Source: CAD feature listing. Evaluate the final solid. Frame: model axes, mm. A direction names the side the tool comes from. Give positions to 0.01 mm unless a question says otherwise; leave off trailing zeros. Loops run counter-clockwise (first coordinate to the right, second up) from the corner with the lowest first, then second, coordinate; pieces in that order, holes last. Notation, with made-up numbers: M -17.5,73.25 L 6.5,73.25 A19 cw 6.5,77.25 Z; hole C 7.5,-20.75 d10. An arc over 180 degrees is marked long. Answer in a Markdown table with one row per item.
```python
from build123d import *

# Parameters (mm, degrees)
SKETCH_3_W           = 180
SKETCH_3_H           = 43
EXTRUDE_1_DEPTH      = 12
CUT_EXTRUDE_1_DEPTH  = 52
CUT_EXTRUDE_2_DEPTH  = 5
CUT_EXTRUDE_3_DEPTH  = 5
SKETCH_8_W           = 55
SKETCH_8_H           = 37
CUT_EXTRUDE_4_DEPTH  = 10.5
CUT_EXTRUDE_5_DEPTH  = 4
SKETCH_10_W          = 62.128790526
SKETCH_10_H          = 8.683746703
CUT_EXTRUDE_6_DEPTH  = 8
CUT_EXTRUDE_8_DEPTH  = 9
FILLET_2_R           = 2
FILLET_3_R           = 3
SKETCH_12_W          = 10
SKETCH_12_H          = 4
CUT_EXTRUDE_9_DEPTH  = 10
SKETCH_13_W          = 4
SKETCH_13_H          = 4
SKETCH_13_H_2        = 7.435323836
SKETCH_13_W_2        = 5
SKETCH_13_H_3        = 5
EXTRUDE_2_DEPTH      = 5
SKETCH_14_W          = 15
SKETCH_14_H          = 1.5
CUT_EXTRUDE_10_DEPTH = 5.5


with BuildPart() as part:
    # 草图3 → 凸台-拉伸1 (new body)
    with BuildSketch(Plane(origin=(0, 0, 0), x_dir=(1, 0, 0), z_dir=(0, 1, 0))):
        with Locations((50.068597249, 7.753123643)):
            Rectangle(SKETCH_3_W, SKETCH_3_H)
    extrude(amount=EXTRUDE_1_DEPTH)

    # 草图4 → 切除-拉伸1 (cut)
    with BuildSketch(Plane(origin=(0, 0, 0), x_dir=(1, 0, 0), z_dir=(0, 1, 0))):
        Polygon((-22.469613434, -5.858946979), (26.002261286, -5.858946979), (29.068597249, -13.746876357), (-25.931402751, -13.746876357), align=None)
    extrude(amount=CUT_EXTRUDE_1_DEPTH, mode=Mode.SUBTRACT)

    # 草图5 → 切除-拉伸2 (cut)
    with BuildSketch(Plane(origin=(0, 12, 0), x_dir=(1, 0, 0), z_dir=(0, 1, 0))):
        Polygon((140.068597249, 7.753123643), (140.068597249, 22.753123643), (125.276479966, 22.753123643), (125.276479966, -7.246876357), (140.068597249, -7.246876357), align=None)
    extrude(amount=-CUT_EXTRUDE_2_DEPTH, mode=Mode.SUBTRACT)

    # 草图7 → 切除-拉伸3 (cut)
    with BuildSketch(Plane(origin=(0, 12, 0), x_dir=(1, 0, 0), z_dir=(0, 1, 0))):
        Polygon((125.276479966, 7.753123643), (125.276479966, 25.753123643), (100.500825538, 25.753123643), (100.500825538, -10.246876357), (125.276479966, -10.246876357), align=None)
    extrude(amount=-CUT_EXTRUDE_3_DEPTH, mode=Mode.SUBTRACT)

    # 草图8 → 切除-拉伸4 (cut)
    with BuildSketch(Plane(origin=(0, 12, 0), x_dir=(1, 0, 0), z_dir=(0, 1, 0))):
        with Locations((63.776287419, 7.753123643)):
            Rectangle(SKETCH_8_W, SKETCH_8_H)
    extrude(amount=-CUT_EXTRUDE_4_DEPTH, mode=Mode.SUBTRACT)

    # 草图9 → 切除-拉伸5 (cut)
    with BuildSketch(Plane(origin=(0, 12, 0), x_dir=(1, 0, 0), z_dir=(0, 1, 0))):
        Polygon((91.276287419, 26.253123643), (96.635770173, 26.253123643), (96.635770173, 22.130591531), (96.635770173, 13.862098754), (97.813575381, 11.877191358), (100.500825538, 11.877191358), (100.500825538, 3.393971617), (96.236747254, 3.393971617), (92.132656028, 10.310430274), (92.132656028, 21.255120764), (91.276287419, 21.255120764), align=None)
    extrude(amount=-CUT_EXTRUDE_5_DEPTH, mode=Mode.SUBTRACT)

    # 草图10 → 切除-拉伸6 (cut)
    with BuildSketch(Plane(origin=(0, 12, 0), x_dir=(1, 0, 0), z_dir=(0, 1, 0))):
        with Locations((1.934159822, -6.405003006)):
            Rectangle(SKETCH_10_W, SKETCH_10_H)
    extrude(amount=-CUT_EXTRUDE_6_DEPTH, mode=Mode.SUBTRACT)

    # 草图11 → 切除-拉伸8 (cut)
    with BuildSketch(Plane(origin=(0, 12, 0), x_dir=(1, 0, 0), z_dir=(0, 1, 0))):
        Polygon((32.998555085, -10.746876357), (-36.5396752, -10.746876357), (-36.5396752, 26.253123643), (36.276287419, 26.253123643), (36.276287419, -2.167243749), (32.998555085, -2.063129654), align=None)
    extrude(amount=-CUT_EXTRUDE_8_DEPTH, mode=Mode.SUBTRACT)

    # 圆角2
    fillet_2_edges = [part.edges().sort_by_distance(p)[0] for p in [
        (84.568597249, 0, 13.746876357),
        (-24.200508092, 0, 9.802911668),
        (27.535429268, 0, 9.802911668),
        (50.068597249, 0, -29.253123643),
        (140.068597249, 0, -7.753123643),
        (-32.931402751, 0, 13.746876357),
        (-39.931402751, 0, -7.753123643),
    ]]
    fillet(fillet_2_edges, radius=FILLET_2_R)

    # 圆角3
    # the kernel refuses this fillet: 3 mm, written as the material it takes off along each edge
    with BuildSketch(Plane(origin=(-36.931402751, 0, 10.746876357), x_dir=(0, 0, 1), z_dir=(1, 0, 0))) as fillet_3_piece_1:
        with BuildLine():
            CenterArc((1, -2), 2, 0, 90)
            Line((3, -2), (3, 0))
            Line((3, 0), (1, 0))
        make_face()
    revolve(axis=Axis((-36.931402751, 0, 10.746876357), (0, -1, 0)), revolution_arc=90, mode=Mode.SUBTRACT)
    with BuildSketch(Plane(origin=(-36.931402751, 0, -26.253123643), x_dir=(-1, 0, 0), z_dir=(0, 0, 1))) as fillet_3_piece_2:
        with BuildLine():
            CenterArc((1, -2), 2, 0, 90)
            Line((3, -2), (3, 0))
            Line((3, 0), (1, 0))
        make_face()
    revolve(axis=Axis((-36.931402751, 0, -26.253123643), (0, -1, 0)), revolution_arc=90, mode=Mode.SUBTRACT)
    with BuildSketch(Plane(origin=(137.068597249, 0, 10.746876357), x_dir=(1, 0, 0), z_dir=(0, 0, -1))) as fillet_3_piece_3:
        with BuildLine():
            CenterArc((1, -2), 2, 0, 90)
            Line((3, -2), (3, 0))
            Line((3, 0), (1, 0))
        make_face()
    revolve(axis=Axis((137.068597249, 0, 10.746876357), (0, -1, 0)), revolution_arc=90, mode=Mode.SUBTRACT)
    with BuildSketch(Plane(origin=(137.068597249, 0, -26.253123643), x_dir=(0, 0, -1), z_dir=(-1, 0, 0))) as fillet_3_piece_4:
        with BuildLine():
            CenterArc((1, -2), 2, 0, 90)
            Line((3, -2), (3, 0))
            Line((3, 0), (1, 0))
        make_face()
    revolve(axis=Axis((137.068597249, 0, -26.253123643), (0, -1, 0)), revolution_arc=90, mode=Mode.SUBTRACT)
    with BuildSketch(Plane(origin=(-39.931402751, 0, -29.253123643), x_dir=(1, 0, 0), z_dir=(0, 1, 0))) as fillet_3_piece_5:
        with BuildLine():
            CenterArc((FILLET_3_R, -FILLET_3_R), FILLET_3_R, 90, 90)
            Line((0, -FILLET_3_R), (0, 0))
            Line((0, 0), (FILLET_3_R, 0))
        make_face()
    extrude(amount=19.5, mode=Mode.SUBTRACT)
    with BuildSketch(Plane(origin=(140.068597249, 0, -29.253123643), x_dir=(-1, 0, 0), z_dir=(0, 1, 0)), Plane(origin=(140.068597249, 0, 13.746876357), x_dir=(0, 0, -1), z_dir=(0, 1, 0)), Plane(origin=(-39.931402751, 0, 13.746876357), x_dir=(1, 0, 0), z_dir=(0, 1, 0))) as fillet_3_piece_6:
        with BuildLine():
            CenterArc((FILLET_3_R, FILLET_3_R), FILLET_3_R, 180, 90)
            Line((0, FILLET_3_R), (0, 0))
            Line((0, 0), (FILLET_3_R, 0))
        make_face()
    extrude(amount=19.5, mode=Mode.SUBTRACT)

    # 草图12 → 切除-拉伸9 (cut)
    with BuildSketch(Plane(origin=(-36.5396752, 0, 0), x_dir=(0, 0, -1), z_dir=(1, 0, 0))):
        with Locations((13.253123643, 10)):
            Rectangle(SKETCH_12_W, SKETCH_12_H)
    extrude(amount=-CUT_EXTRUDE_9_DEPTH, mode=Mode.SUBTRACT)

    # 草图13 → 凸台-拉伸2 (add)
    with BuildSketch(Plane(origin=(0, 3, 0), x_dir=(1, 0, 0), z_dir=(0, 1, 0))):
        with Locations((-34.5396752, 24.253123643)):
            Rectangle(SKETCH_13_W, SKETCH_13_H)
        with Locations((-34.5396752, 4.535461725)):
            Rectangle(SKETCH_13_W, SKETCH_13_H_2)
        with Locations((-10.5396752, 24.253123643)):
            Rectangle(SKETCH_13_W, SKETCH_13_H)
        with Locations((-0.0396752, 4.753123643)):
            Rectangle(SKETCH_13_W_2, SKETCH_13_H_3)
    extrude(amount=EXTRUDE_2_DEPTH)

    # 草图14 → 切除-拉伸10 (cut)
    with BuildSketch(Plane(origin=(0, 12, 0), x_dir=(1, 0, 0), z_dir=(0, 1, 0))):
        with Locations((28.776287419, 27.003123643)):
            Rectangle(SKETCH_14_W, SKETCH_14_H)
    extrude(amount=-CUT_EXTRUDE_10_DEPTH, mode=Mode.SUBTRACT)


solid = part.part
```
Q1. Section query B-B (x = 66.5). Output: boundary loops of the cut face in (y, z).
Values follow:
| item | result |
|---|---|
| outline | M 0,-27.25 A2 ccw 2,-29.25 L 12,-29.25 L 12,-26.25 L 1.5,-26.25 L 1.5,10.75 L 12,10.75 L 12,13.75 L 2,13.75 A2 ccw 0,11.75 Z |
Q2. Ray query, probe 1 along Z at (x, y) = (40, 7); probe 2 along X at (y, z) = (7.75, -3.5); probe 3 along X at (y, z) = (9.25, 1). Return the intervals inside material, ascending. Write a range as from..to.
Values follow:
| item | result |
|---|---|
| probe 1 | -29.25..-26.25, 10.75..13.75 |
| probe 2 | -39.93..-32.54, -2.54..2.46, 91.28..100.5 |
| probe 3 | -39.93..-36.54, 91.28..100.5 |
Q3. Section query A-A (z = -16.5). Output: boundary loops of the cut face in (x, y).
Values follow:
| item | result |
|---|---|
| outline | M -39.93,2 A2 ccw -37.93,0 L 138.07,0 A2 ccw 140.07,2 L 140.07,7 L 100.5,7 L 100.5,12 L 96.64,12 L 96.64,8 L 92.13,8 L 92.13,12 L 91.28,12 L 91.28,1.5 L 36.28,1.5 L 36.28,3 L -36.54,3 L -36.54,8 L -39.93,8 Z |
Q4. Reachability of faces 4 (the flat face through (29, 9, -27.753)), 5 (the flat face through (-38, 8, -13)), 6 (the flat face through (-11, 5, -22.253)), 7 (the flat face through (133, 10, -22.753)) from +Z, -Z, +X, -X, +Y, -Y: full face, straight path, thin tool, end or side. Return the list, or none.
Values follow:
| item | result |
|---|---|
| face 4 | +Y |
| face 5 | -X, +Y |
| face 6 | +Z, +Y |
| face 7 | +X, +Y |
Q5. Section query C-C (y = 10.25). Give the number of separate pieces and of enclosed holes in the cut face, plus the area to 3 significant figures.
Values follow:
| item | result |
|---|---|
| separate pieces | 3 |
| enclosed holes | 0 |
| area | 1,350 mm^2 |
Q6. Section query D-D (x = 23). Output: boundary loops of the cut face in (y, z).
Values follow:
| item | result |
|---|---|
| outline | M 0,-27.25 A2 ccw 2,-29.25 L 12,-29.25 L 12,-27.75 L 6.5,-27.75 L 6.5,-26.25 L 3,-26.25 L 3,5.86 L 0,5.86 Z |
Q7. Mould query, pull axis X, two halves, no side actions, for faces 1 (the cylindrical face through (-39.08, 6.93, 12.84)), 2 (the flat face through (-32, 7, 13.747)), 3 (the flat face through (-35, 5, -0.818)). Classes: +X half, -X half, draft (parallel to the pull), parting line (faces both ways), or undercut.
Values follow:
| item | result |
|---|---|
| face 1 | -X half |
| face 2 | draft |
| face 3 | undercut |
Q8. Contact query for flat-ended pins moving along their axis: pin 1 Ø1.2 at (x, z) = (-34.5, -25) entering from +Y; pin 2 Ø11 at (x, z) = (-17.5, -7.5) entering from +Y; pin 3 Ø3 at (x, y) = (-11.5, 6.5) entering from +Z. Output: stop coordinate, or through.
Values follow:
| item | result |
|---|---|
| pin 1 | y = 8 |
| pin 2 | y = 3 |
| pin 3 | z = -22.25 |
